Build history of the part. All positions in model axes, mm. A direction names the side the tool comes from. Give positions to 0.01 mm unless a question says otherwise; leave off trailing zeros. Loops run counter-clockwise (first coordinate to the right, second up) from the corner with the lowest first, then second, coordinate; pieces in that order, holes last. Notation, with made-up numbers: (46, 50.5) -> (79, 50.5) arc R19 ccw to (79, 79.5) -> close; hole circle Ø3 at (39.25, 6). An arc over 180 degrees is marked (long way). Answer as a JSON object with one key per item and string values. Group by question number.
Q1. Wall check: probe 1 along X at (y, z) = (4, 1.35); probe 2 along Y at (x, z) = (-3.5, 1.05); probe 3 along Z at (x, y) = (11, 6.5). Give the ranges that are in metal, low to high. Write a range as from..to.
Q2. Tool access for faces 1 (the flat face through (0, -5.85, 1)), 2 (the flat face through (-14.85, 0, 1)), 3 (the flat face through (0, 5.85, 1)): list every direction of +Z, -Z, +X, -X, +Y, -Y with a clear straight run to the whole face (end or side of a thin tool).
Q3. Drop flat-ended pins along their axis: pin 1 (0.8 mm diameter, centred on x = 4, z = 1, fed in from -Y); pin 2 (0.8 mm diameter, centred on y = 1, z = 1, fed in from +X); pin 3 (8 mm diameter, centred on x = 9, y = 5, fed in from -Z); pin 4 (0.5 mm diameter, centred on x = -3.5, z = 1, fed in from +Y). Give the stop position or say it passes through.
Q4. Band-saw the part on A-A, the plane x = 3.5. Write the cut outline in (y, z), plus the area to 3 significant figures.
Q5. Band-saw the part on B-B, the plane z = 0.95. Write the cut outline in (x, y).
Q6. Band-saw the part on C-C, the plane y = 6.25. Write the cut outline in (x, z), plus the area to 3 significant figures.
from build123d import *

# Parameters (mm, degrees)
SKETCH_W     = 33
SKETCH_H     = 15
PAD_DEPTH    = 0.5
SKETCH001_W  = 29.7
SKETCH001_H  = 11.7
PAD001_DEPTH = 1
FILLET_R     = 0.5


with BuildPart() as part:
    # Sketch → Pad (new body)
    with BuildSketch(Plane.XY):
        Rectangle(SKETCH_W, SKETCH_H)
    extrude(amount=PAD_DEPTH)

    # Sketch001 (on Face6 of Pad) → Pad001 (join)
    with BuildSketch(Plane.XY.offset(0.5)):
        Rectangle(SKETCH001_W, SKETCH001_H)
    extrude(amount=PAD001_DEPTH)

    # Fillet
    fillet_edges = [part.edges().sort_by_distance(p)[0] for p in [
        (-14.85, -5.85, 1),
        (14.85, -5.85, 1),
        (14.85, 5.85, 1),
        (-14.85, 5.85, 1),
    ]]
    fillet(fillet_edges, radius=FILLET_R)


solid = part.part
Worked answers:
{
 "1": {"probe 1": "-14.85..14.85", "probe 2": "-5.85..5.85", "probe 3": "0..0.5"},
 "2": {"face 1": "+Z, +X, -X, -Y", "face 2": "+Z, -X, +Y, -Y", "face 3": "+Z, +X, -X, +Y"},
 "3": {"pin 1": "y = -5.85", "pin 2": "x = 14.85", "pin 3": "z = 0", "pin 4": "y = 5.85"},
 "4": {"outline": "(-7.5, 0) -> (7.5, 0) -> (7.5, 0.5) -> (5.85, 0.5) -> (5.85, 1.5) -> (-5.85, 1.5) -> (-5.85, 0.5) -> (-7.5, 0.5) -> close", "area": "19.2 mm2"},
 "5": {"outline": "(-14.85, -5.35) arc R0.5 ccw to (-14.35, -5.85) -> (14.35, -5.85) arc R0.5 ccw to (14.85, -5.35) -> (14.85, 5.35) arc R0.5 ccw to (14.35, 5.85) -> (-14.35, 5.85) arc R0.5 ccw to (-14.85, 5.35) -> close"},
 "6": {"outline": "(-16.5, 0) -> (16.5, 0) -> (16.5, 0.5) -> (-16.5, 0.5) -> close", "area": "16.5 mm2"}
}
